Part model, mm, in its own coordinate system. A direction names the side the tool comes from. Give positions to 0.01 mm unless a question says otherwise; leave off trailing zeros. Order: outer loops, then holes, each group sorted by start corner. A loop starts at its lowest first (then second) coordinate and runs counter-clockwise, first axis right, second up. Notation, with made-up numbers: (15.25, 22.25) - (73.25, 22.25) arc R23 ccw to (73.25, 30.25) - close; hole circle Ø4 at (-23, 43.25). An arc over 180 degrees is marked (long way). Use one line per item in the form item = value. Start each with the question number.
1. Band-saw the part on A-A, the plane y = 4.25. List the corners of the cut face in (x, z), plus the area to 3 significant figures.
2. Pin check, flat tips, straight feed: P1, Ø0.5, axis at x = 22.5, y = 1, coming from the +Z side; P2, Ø1.4, axis at y = 9, z = 1.5, coming from the +X side; P3, Ø1.6, axis at y = 15.5, z = 2, coming from the -X side. Stop position of each tip, or through.
3. Band-saw the part on B-B, the plane z = 1.3. List the corners of the cut face in (x, y), plus the area to 3 significant figures.
4. Drill centre lines: line 1 (X direction, y = 8, z = 2.15); line 2 (X direction, y = 14.25, z = 0.45); line 3 (Y direction, x = 20, z = 2.3). Where is each one in solid material? Low to high.
5. Tool access for faces 1 (the face through (6.866, 11, 1)), 2 (the face through (33.23, 12.14, 1.71)), 3 (the face through (33.23, 10.86, 1.69)), 4 (the face through (19, 1, 2.2)): list every direction of +Z, -Z, +X, -X, +Y, -Y with a clear straight run to the whole face (end or side of a thin tool).
6. Pull direction Y, two halves, no side cores. Call faces 5 (the face through (34.066, -1, 1)), 6 (the face through (32.866, 5, 2)), 7 (the face through (19, 23, 2)): +Y half, -Y half, draft (parallel to the pull), parting line (faces both ways), or undercut.
7. Band-saw the part on C-C, the plane x = 10. List the corners of the cut face in (y, z), plus the area to 3 significant figures.
from build123d import *

# Parameters (mm, degrees)
SKIZZE1_W                       = 28
SKIZZE1_H                       = 23
AUFSATZ_LINEAR_AUSTRAGEN1_DEPTH = 0.7
SKIZZE3_W                       = 27
SKIZZE3_H                       = 22.5
AUFSATZ_LINEAR_AUSTRAGEN2_DEPTH = 2
AUFSATZ_LINEAR_AUSTRAGEN4_DEPTH = 1.7
SKIZZE6_W                       = 0.6
SKIZZE6_H                       = 22
SCHNITT_LINEAR_AUSTRAGEN1_DEPTH = 10
SKIZZE7_W                       = 2
SKIZZE7_H                       = 2
AUFSATZ_LINEAR_AUSTRAGEN5_DEPTH = 0.5
SKIZZE8_W                       = 2
SKIZZE8_H                       = 2
AUFSATZ_LINEAR_AUSTRAGEN6_DEPTH = 0.5
VERRUNDUNG1_R                   = 1
VERRUNDUNG2_R                   = 1
SKIZZE9_W                       = 27
SKIZZE9_H                       = 2.5
AUFSATZ_LINEAR_AUSTRAGEN7_DEPTH = 2.7
SKIZZE10_W                      = 28
SKIZZE10_H                      = 0.7
AUFSATZ_LINEAR_AUSTRAGEN8_DEPTH = 0.5
SKIZZE11_W                      = 19.4
SKIZZE11_H                      = 1
SCHNITT_LINEAR_AUSTRAGEN2_DEPTH = 0.5


with BuildPart() as part:
    # Skizze1 → Aufsatz-Linear austragen1 (new body)
    with BuildSketch(Plane.XY):
        with Locations((19.366132402, 11.5)):
            Rectangle(SKIZZE1_W, SKIZZE1_H)
    extrude(amount=AUFSATZ_LINEAR_AUSTRAGEN1_DEPTH)

    # Skizze3 → Aufsatz-Linear austragen2 (add)
    with BuildSketch(Plane.XY.offset(0.7)):
        with Locations((19.366132402, 11.25)):
            Rectangle(SKIZZE3_W, SKIZZE3_H)
    extrude(amount=AUFSATZ_LINEAR_AUSTRAGEN2_DEPTH)

    # Skizze5 → Aufsatz-Linear austragen4 (add)
    with BuildSketch(Plane.XZ):
        Polygon((5.866132402, 2.7), (32.866132402, 2.7), (34.066132402, 2.7), (34.066132402, 0), (33.366132402, 0), (5.366132402, 0), (4.666132402, 0), (4.666132402, 2.7), align=None)
    extrude(amount=AUFSATZ_LINEAR_AUSTRAGEN4_DEPTH)

    # Skizze6 → Schnitt-Linear austragen1 (cut)
    with BuildSketch(Plane(origin=(0, 0, 0), x_dir=(-1, 0, 0), z_dir=(0, 0, -1))):
        with Locations((-31.466132402, 12)):
            Rectangle(SKIZZE6_W, SKIZZE6_H)
        with Locations((-7.166132402, 12)):
            Rectangle(SKIZZE6_W, SKIZZE6_H)
    extrude(amount=-SCHNITT_LINEAR_AUSTRAGEN1_DEPTH, mode=Mode.SUBTRACT)

    # Skizze7 → Aufsatz-Linear austragen5 (add)
    with BuildSketch(Plane(origin=(32.866132402, 0, 0), x_dir=(0, 0, -1), z_dir=(1, 0, 0))):
        with Locations((-1.7, 11.5)):
            Rectangle(SKIZZE7_W, SKIZZE7_H)
    extrude(amount=AUFSATZ_LINEAR_AUSTRAGEN5_DEPTH)

    # Skizze8 → Aufsatz-Linear austragen6 (add)
    with BuildSketch(Plane.ZY.offset(-5.866132402)):
        with Locations((1.7, 11.5)):
            Rectangle(SKIZZE8_W, SKIZZE8_H)
    extrude(amount=AUFSATZ_LINEAR_AUSTRAGEN6_DEPTH)

    # Verrundung1
    # the kernel refuses this fillet: 1 mm, written as the material it takes off along each edge
    with BuildSketch(Plane(origin=(33.366132402, 10.5, 0.7), x_dir=(-1, 0, 0), z_dir=(0, 0, 1))) as verrundung1_piece_1:
        with BuildLine():
            CenterArc((1, -0.866025404), VERRUNDUNG1_R, 120, 60)
            Line((0, -0.866025404), (0, 0))
            Line((0, 0), (0.5, 0))
        make_face()
    extrude(amount=4.165063509, mode=Mode.SUBTRACT)
    with BuildSketch(Plane(origin=(33.366132402, 12.5, 4.865063509), x_dir=(0, -1, 0), z_dir=(0, 0, -1))) as verrundung1_piece_2:
        with BuildLine():
            CenterArc((0.866025404, 1), VERRUNDUNG1_R, 210, 60)
            Line((0, 0.5), (0, 0))
            Line((0, 0), (0.866025404, 0))
        make_face()
    extrude(amount=4.165063509, mode=Mode.SUBTRACT)

    # Verrundung2
    # the kernel refuses this fillet: 1 mm, written as the material it takes off along each edge
    with BuildSketch(Plane(origin=(5.366132402, 12.5, 0.7), x_dir=(1, 0, 0), z_dir=(0, 0, 1))) as verrundung2_piece_1:
        with BuildLine():
            CenterArc((1, -0.866025404), VERRUNDUNG2_R, 120, 60)
            Line((0, -0.866025404), (0, 0))
            Line((0, 0), (0.5, 0))
        make_face()
    extrude(amount=4.165063509, mode=Mode.SUBTRACT)
    with BuildSketch(Plane(origin=(5.366132402, 10.5, 4.865063509), x_dir=(0, 1, 0), z_dir=(0, 0, -1))) as verrundung2_piece_2:
        with BuildLine():
            CenterArc((0.866025404, 1), VERRUNDUNG2_R, 210, 60)
            Line((0, 0.5), (0, 0))
            Line((0, 0), (0.866025404, 0))
        make_face()
    extrude(amount=4.165063509, mode=Mode.SUBTRACT)

    # Skizze9 → Aufsatz-Linear austragen7 (add)
    with BuildSketch(Plane.XY.offset(2.7)):
        with Locations((19.366132402, 21.75)):
            Rectangle(SKIZZE9_W, SKIZZE9_H)
    extrude(amount=-AUFSATZ_LINEAR_AUSTRAGEN7_DEPTH)

    # Skizze10 → Aufsatz-Linear austragen8 (add)
    with BuildSketch(Plane(origin=(0, 23, 0), x_dir=(1, 0, 0), z_dir=(0, 1, 0))):
        with Locations((19.366132402, -0.35)):
            Rectangle(SKIZZE10_W, SKIZZE10_H)
    extrude(amount=AUFSATZ_LINEAR_AUSTRAGEN8_DEPTH)

    # Skizze11 → Schnitt-Linear austragen2 (cut)
    with BuildSketch(Plane.XY.offset(2.7)):
        with Locations((19.366132402, 0.8)):
            Rectangle(SKIZZE11_W, SKIZZE11_H)
    extrude(amount=-SCHNITT_LINEAR_AUSTRAGEN2_DEPTH, mode=Mode.SUBTRACT)


solid = part.part
From the geometry:
q1.outline = (5.37, 0) - (6.87, 0) - (6.87, 2.7) - (5.87, 2.7) - (5.87, 0.7) - (5.37, 0.7) - close; (7.47, 0) - (31.17, 0) - (31.17, 2.7) - (7.47, 2.7) - close; (31.77, 0) - (33.37, 0) - (33.37, 0.7) - (32.87, 0.7) - (32.87, 2.7) - (31.77, 2.7) - close
q1.area = 70.4 mm²
q2.P1 = 2.2
q2.P2 = 32.87
q2.P3 = 5.87
q3.outline = (4.67, -1.7) - (34.07, -1.7) - (34.07, 0) - (32.87, 0) - (32.87, 10.5) arc R1 ccw to (33.37, 11.37) - (33.37, 11.63) arc R1 ccw to (32.87, 12.5) - (32.87, 23) - (5.87, 23) - (5.87, 12.5) arc R1 ccw to (5.37, 11.63) - (5.37, 11.37) arc R1 ccw to (5.87, 10.5) - (5.87, 0) - (4.67, 0) - close; hole (6.87, 1) - (7.47, 1) - (7.47, 20.5) - (6.87, 20.5) - close; hole (31.17, 1) - (31.77, 1) - (31.77, 20.5) - (31.17, 20.5) - close
q3.area = 649 mm²
q4.line_1 = 5.87 to 6.87, 7.47 to 31.17, 31.77 to 32.87
q4.line_2 = 5.37 to 6.87, 7.47 to 31.17, 31.77 to 33.37
q4.line_3 = -1.7 to 0.3, 1.3 to 23
q5.face_1 = +Z, -Z
q5.face_2 = +Z, +X, +Y
q5.face_3 = +Z, +X
q5.face_4 = +Z
q6.face_5 = draft
q6.face_6 = undercut
q6.face_7 = +Y half
q7.outline = (-1.7, 0) - (23.5, 0) - (23.5, 0.7) - (23, 0.7) - (23, 2.7) - (1.3, 2.7) - (1.3, 2.2) - (0.3, 2.2) - (0.3, 2.7) - (-1.7, 2.7) - close
q7.area = 66.5 mm²
